```python
from build123d import *

# Parameters (mm, degrees)
F0_W     = 128.016
F0_H     = 22.352
F1_DEPTH = 66.548


with BuildPart() as f1:
    # F0 (on Front) → F1 (new body)
    with BuildSketch(Plane.XZ):
        Polygon((-44.265021, 16.786693), (-66.617021, 16.786693), (-66.617021, -46.713307), (-44.265021, -46.713307), (-44.265021, -24.361307), align=None)
        with Locations((19.742979, -35.537307)):
            Rectangle(F0_W, F0_H)
        Polygon((106.102979, -24.361307), (83.750979, -24.361307), (83.750979, -46.713307), (83.750979, -65.509307), (106.102979, -65.509307), align=None)
    extrude(amount=-F1_DEPTH)


solid = f1.part
```
Geometry: final body of the model. Coordinates: model frame, mm. A direction names the side the tool comes from. Give positions to 0.01 mm unless a question says otherwise; leave off trailing zeros. Order: outer loops, then holes, each group sorted by start corner. A loop starts at its lowest first (then second) coordinate and runs counter-clockwise, first axis right, second up. Notation, with made-up numbers: M -4.5,-40 L 13.5,-40 A33 cw 13.5,-9 Z; hole C 45.5,14.5 d3. An arc over 180 degrees is marked long. Answer as CSV lines item,"result". Start each with the question number.
1) Cut plane C-C (x = 54). Output: boundary loops of the cut face in (y, z), then the cut area to 3 significant figures.
2) First-contact query: P1, Ø10, axis at x = -28, y = 51.5, coming from the +Z side; P2, Ø15, axis at y = 23, z = -58, coming from the -X side. Flat tips, straight axial feed; report the tip coordinate or a pass-through.
3) Cut plane B-B (z = -59). Output: boundary loops of the cut face in (x, y), then the cut area to 3 significant figures.
4) Set-up query: faces 1 (the flat face through (32, 33, -24.361)), 2 (the flat face through (106.103, 33, -45)), 3 (the flat face through (8, 33, -46.713)). Return all of +Z, -Z, +X, -X, +Y, -Y with unobstructed straight access to the full face (end or side cutting, diameter ignored); none if empty.
5) Cut plane A-A (y = 33.5). Output: boundary loops of the cut face in (x, z), then the cut area to 3 significant figures.
6) Line query: line 1 (X direction, y = 25.5, z = -18.5); line 2 (Z direction, x = 50, y = 21.5); line 3 (Z direction, x = 98, y = 36). Output: solid intervals per line, ascending. Write a range as from..to.
Findings below:
1,outline,"M 0,-46.71 L 66.55,-46.71 L 66.55,-24.36 L 0,-24.36 Z"
1,area,"1,490 mm²"
2,P1,"stops at z = -24.36"
2,P2,"stops at x = 83.75"
3,outline,"M 83.75,0 L 106.1,0 L 106.1,66.55 L 83.75,66.55 Z"
3,area,"1,490 mm²"
4,face 1,"+Z, +X, +Y, -Y"
4,face 2,"+Z, -Z, +X, +Y, -Y"
4,face 3,"-Z, -X, +Y, -Y"
5,outline,"M -66.62,-46.71 L 83.75,-46.71 L 83.75,-65.51 L 106.1,-65.51 L 106.1,-24.36 L -44.27,-24.36 L -44.27,16.79 L -66.62,16.79 Z"
5,area,"5,200 mm²"
6,line 1,"x = -66.62..-44.27"
6,line 2,"z = -46.71..-24.36"
6,line 3,"z = -65.51..-24.36"
